from build123d import *

# Parameters (mm, degrees)
BOSS_EXTRUDE1_DEPTH = 25
SKETCH2_W           = 1
SKETCH2_H           = 1
CUT_EXTRUDE1_DEPTH  = 15
BOSS_EXTRUDE2_DEPTH = 3
LPATTERN1_COUNT     = 21
LPATTERN1_PITCH     = 0.71


with BuildPart() as part:
    # Sketch1 → Boss-Extrude1 (new body)
    with BuildSketch(Plane(origin=(0, 0, 0), x_dir=(1, 0, 0), z_dir=(0, 1, 0))):
        Polygon((2, 4), (-2, 4), (-2, 3), (-1, 3), (-1, 0), (1, 0), (1, 3), (2, 3), align=None)
    boss_extrude1 = extrude(amount=BOSS_EXTRUDE1_DEPTH)

    # Mirror1: Boss-Extrude1 across plane
    add(boss_extrude1.mirror(Plane(origin=(-1, 25, 0), x_dir=(1, 0, 0), z_dir=(0, 0, -1))))

    # Sketch2 → Cut-Extrude1 (cut)
    with BuildSketch(Plane(origin=(0, 25, 0), x_dir=(1, 0, 0), z_dir=(0, 1, 0))):
        with Locations((-1.5, -3.5)):
            Rectangle(SKETCH2_W, SKETCH2_H)
    extrude(amount=-CUT_EXTRUDE1_DEPTH, mode=Mode.SUBTRACT)

    # Sketch3 → Boss-Extrude2 (add)
    with BuildSketch(Plane.XY.offset(4)):
        Polygon((-1, 10), (-2, 10.355), (-1, 10.71), align=None)
    boss_extrude2 = extrude(amount=-BOSS_EXTRUDE2_DEPTH)

    # LPattern1: Boss-Extrude2 ×21
    with Locations(*[(0, i * LPATTERN1_PITCH, 0) for i in range(1, LPATTERN1_COUNT)]):
        add(boss_extrude2)


solid = part.part
The model under review builds one solid part; all positions refer to its coordinate system, in mm. A direction names the side the tool comes from. Coordinates: 2 decimals unless noted, no trailing zeros. Loops run counter-clockwise (first coordinate to the right, second up) from the corner with the lowest first, then second, coordinate; pieces in that order, holes last. Notation, with made-up numbers: (-20, 53) -> (0, 53) arc R27 cw to (0, 77) -> close; hole circle Ø1 at (72, 13). An arc over 180 degrees is marked (long way). Use a Markdown table: item, result. Add a question column.
1. Add section D-D on x = -1.7. Give the number of separate pieces and of enclosed holes in the cut face, plus the area to 3 significant figures.
2. Machinability: for faces 1 (the face through (-1.5, 12.3, -3)), 2 (the face through (-1.5, 4.9, 3)), 3 (the face through (2, 12.3, 3.5)), 4 (the face through (-2, 4.9, 3.5)), 5 (the face through (1.5, 12.3, 3)), which of the approach directions +Z, -Z, +X, -X, +Y, -Y give a long, thin tool a straight path to every point of the face, cutting with its end or side? Answer none if there is none.
3. Add section C-C on z = -1.5. Write out the cut boundary in (x, y).
4. Add section A-A on y = 8.5. Write out the cut boundary in (x, z), plus the area to 3 significant figures.
5. Draft analysis for pull direction Y (two halves, no side actions). For faces 6 (the face through (-1.51, 24.73, 2.52)), 7 (the face through (-1.493, 13.725, 2.521)), 8 (the face through (-1.51, 11.24, 2.52)), 9 (the face through (-1, 10, 0)), state which applies: pulls with the +Y half, pulls with the -Y half, needs draft (parallel to the pull), parting line crosses it, or undercut.
6. Clearance check with flat-ended pins moving along their axes: pin 1 Ø0.5 at (x, z) = (-1.5, 3.5) entering from +Y; pin 2 Ø3 at (y, z) = (10.5, 1) entering from +X; pin 3 Ø1.5 at (y, z) = (21, 2.5) entering from -X. State where each tip first meets the part, or that it passes through.
7. Add section B-B on x = 1.4. Write out the cut boundary in (y, z), plus the area to 3 significant figures.
8. To check wall thickness, follow line 1 (Z direction, x = 1.75, y = 10); line 2 (X direction, y = 10.75, z = -1.5). State the ranges of each line that lie inside material, in increasing order.
Returned:
| question | item | result |
|---|---|---|
| 1 | separate pieces | 23 |
| 1 | enclosed holes | 0 |
| 1 | area | 48.4 mm² |
| 2 | face 1 | -X, +Y, -Y |
| 2 | face 2 | -X, -Y |
| 2 | face 3 | +Z, -Z, +X, +Y, -Y |
| 2 | face 4 | +Z, -Z, -X, +Y, -Y |
| 2 | face 5 | +X, +Y, -Y |
| 3 | outline | (-1, 0) -> (1, 0) -> (1, 25) -> (-1, 25) -> close |
| 4 | outline | (-2, -4) -> (2, -4) -> (2, -3) -> (1, -3) -> (1, 3) -> (2, 3) -> (2, 4) -> (-2, 4) -> (-2, 3) -> (-1, 3) -> (-1, -3) -> (-2, -3) -> close |
| 4 | area | 20.0 mm² |
| 5 | face 6 | pulls with the +Y half |
| 5 | face 7 | undercut |
| 5 | face 8 | undercut |
| 5 | face 9 | needs draft |
| 6 | pin 1 | stops at y = 24.82 |
| 6 | pin 2 | stops at x = 1 |
| 6 | pin 3 | stops at x = -2 |
| 7 | outline | (0, -4) -> (25, -4) -> (25, -3) -> (0, -3) -> close; (0, 3) -> (25, 3) -> (25, 4) -> (0, 4) -> close |
| 7 | area | 50.0 mm² |
| 8 | line 1 | z = -4 to -3, 3 to 4 |
| 8 | line 2 | x = -1 to 1 |
